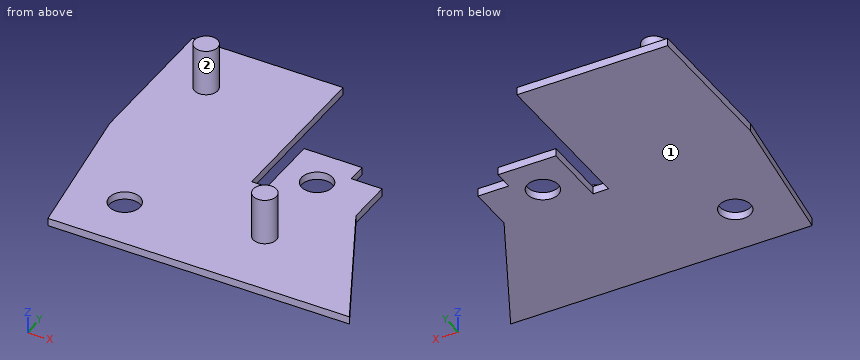
from build123d import *

# Parameters (mm, degrees)
PAD_DEPTH    = 1
SKETCH001_R  = 1.5
PAD001_DEPTH = 6
SKETCH002_R  = 2
POCKET_DEPTH = 1.001


with BuildPart() as part:
    # Sketch → Pad (new body)
    with BuildSketch(Plane.XY):
        Polygon((0, 0), (39, 0), (30, 17.5), (30, 23.5), (26, 23.5), (26, 26), (18.5, 26), (18.5, 17.5), (16.5, 17.5), (16.5, 38.5), (-3, 38.5), (-3, 19.5), align=None)
    extrude(amount=PAD_DEPTH)

    # Sketch001 (on Face14 of Pad) → Pad001 (join)
    with BuildSketch(Plane.XY.offset(1)):
        with Locations((3, 31)):
            Circle(SKETCH001_R)
        with Locations((23, 9)):
            Circle(SKETCH001_R)
    extrude(amount=PAD001_DEPTH)

    # Sketch002 (on Face5 of Pad001) → Pocket (cut, through all)
    with BuildSketch(Plane.XY.offset(1)):
        with Locations((6, 7)):
            Circle(SKETCH002_R)
        with Locations((23, 21)):
            Circle(SKETCH002_R)
    extrude(amount=-POCKET_DEPTH, mode=Mode.SUBTRACT)


solid = part.part
For this review, take the finished solid that the model builds, in its own axes (mm). Face numbers are marked on the shaded views. A direction names the side the tool comes from. Give positions to 0.01 mm unless a question says otherwise; leave off trailing zeros. Order: outer loops, then holes, each group sorted by start corner. A loop starts at its lowest first (then second) coordinate and runs counter-clockwise, first axis right, second up. Notation, with made-up numbers: (22.25, 38.5) - (56.25, 38.5) arc R28 ccw to (56.25, 64.5) - close; hole circle Ø7 at (-16, 22.25). An arc over 180 degrees is marked (long way). Answer as a JSON object with one key per item and string values. Group by question number.
Item 1: Wall thickness on line 1 along Y through (x, z) = (23, 0.7); line 2 along Z through (x, y) = (23, 3); line 3 along X through (y, z) = (30, 3): over which ranges is each line inside the solid? List them lowest first.
Item 2: Take a section at B-B on y = 31. Give the boundary of the cut face in (x, z).
Item 3: Machinability: for the marked faces 1 and 2, which of the approach directions +Z, -Z, +X, -X, +Y, -Y give a long, thin tool a straight path to every point of the face, cutting with its end or side? Answer none if there is none.
Item 4: Take a section at C-C on x = 3. Give the boundary of the cut face in (y, z), and give its area (3 significant figures).
Item 5: Take a section at A-A on y = 21. Give the boundary of the cut face in (x, z), and give its area (3 significant figures).
Item 6: Clearance check with flat-ended pins moving along their axes: pin 1 Ø0.5 at (x, z) = (23, 0.5) entering from +Y; pin 2 Ø5 at (x, y) = (13.5, 31.5) entering from +Z; pin 3 Ø0.8 at (x, z) = (28, 0.5) entering from +Y; pin 4 Ø1 at (x, y) = (21.5, 4) entering from -Z. State where each tip first meets the part, or that it passes through.
Item 7: Take a section at D-D on z = 2.75. Give the boundary of the cut face in (x, y).
Reported:
{
 "1": {"line 1": "0 to 19, 23 to 26", "line 2": "0 to 1", "line 3": "1.88 to 4.12"},
 "2": {"outline": "(-3, 0) - (16.5, 0) - (16.5, 1) - (4.5, 1) - (4.5, 7) - (1.5, 7) - (1.5, 1) - (-3, 1) - close"},
 "3": {"face 1": "-Z, +X, -X, +Y, -Y", "face 2": "+Z"},
 "4": {"outline": "(0, 0) - (38.5, 0) - (38.5, 1) - (32.5, 1) - (32.5, 7) - (29.5, 7) - (29.5, 1) - (0, 1) - close", "area": "56.5 mm^2"},
 "5": {"outline": "(-3, 0) - (16.5, 0) - (16.5, 1) - (-3, 1) - close; (18.5, 0) - (21, 0) - (21, 1) - (18.5, 1) - close; (25, 0) - (30, 0) - (30, 1) - (25, 1) - close", "area": "27.0 mm^2"},
 "6": {"pin 1": "y = 26", "pin 2": "z = 1", "pin 3": "y = 23.5", "pin 4": "z = 0"},
 "7": {"outline": "circle Ø3 at (3, 31); circle Ø3 at (23, 9)"}
}
